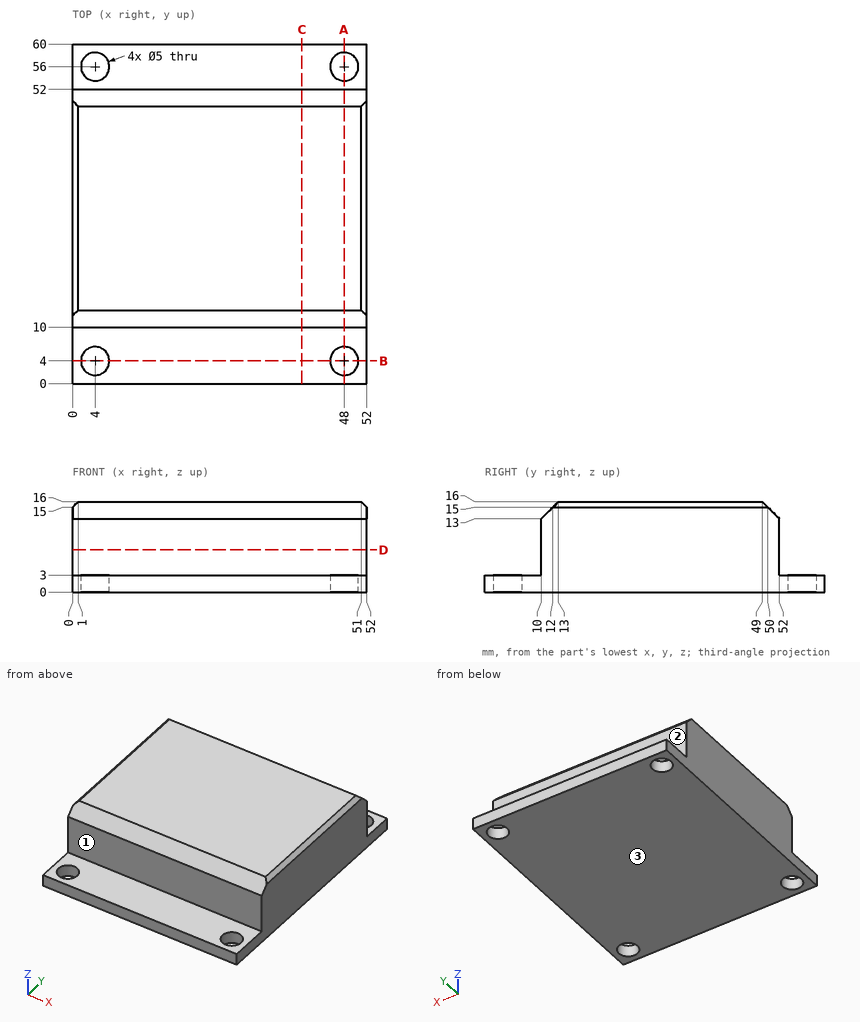
Can you work these out from the drawing? Everything is in mm from the part's minimum corner. A direction names the side the tool comes from. Give positions to 0.01 mm unless a question says otherwise; leave off trailing zeros. Loops run counter-clockwise (first coordinate to the right, second up) from the corner with the lowest first, then second, coordinate; pieces in that order, holes last. Notation, with made-up numbers: M -11.5,46.5 L 24.5,46.5 A26 cw 24.5,62.5 Z; hole C 36,-30 d8. An arc over 180 degrees is marked long. Use CSV: the item, a comma, the result in double quotes. Start each with the question number.
1. On a 3-axis mill with a long thin cutter (end or side, diameter ignored), from which of +Z, -Z, +X, -X, +Y, -Y can I reach the whole of each face in a straight line? I mean the marked faces 1, 2 and 3. Say none if no direction works.
2. Imagine slicing it at D-D, the plane z = 7.5. Write out the boundary of the cut face in (x, y).
3. If I drill on L1, parallel to Y at x = 4, z = 1.75; L2, parallel to Y at x = 27.5, z = 10.75; L3, parallel to Z at x = 46.5, y = 50, over which ranges is the centre line in solid material (lowest first)?
4. Imagine slicing it at C-C, the plane x = 40.5. Write out the boundary of the cut face in (y, z), plus the area to 3 significant figures.
5. Imagine slicing it at A-A, the plane x = 48. Write out the boundary of the cut face in (y, z).
6. Imagine slicing it at B-B, the plane y = 4. Write out the boundary of the cut face in (x, z), plus the area to 3 significant figures.
7. For P1, Ø3, axis at x = 23, y = 3.5, coming from the +Z side; P2, Ø3, axis at x = 36.5, z = 7, coming from the -Y side, each with a flat end and sliding along its axis, tell me the tip position at first contact or that it passes through.
Response values:
1,face 1,"+Z, +X, -X, -Y"
1,face 2,"+Z, +X, -X, +Y"
1,face 3,"-Z, +X, -X, +Y, -Y"
2,outline,"M 0,10 L 52,10 L 52,52 L 0,52 Z"
3,L1,"0 to 1.5, 6.5 to 53.5, 58.5 to 60"
3,L2,"10 to 52"
3,L3,"0 to 15"
4,outline,"M 0,0 L 60,0 L 60,3 L 52,3 L 52,13 L 49,16 L 13,16 L 10,13 L 10,3 L 0,3 Z"
4,area,"717 mm^2"
5,outline,"M 0,0 L 1.5,0 L 1.5,3 L 0,3 Z; M 6.5,0 L 53.5,0 L 53.5,3 L 52,3 L 52,13 L 49,16 L 13,16 L 10,13 L 10,3 L 6.5,3 Z; M 58.5,0 L 60,0 L 60,3 L 58.5,3 Z"
6,outline,"M 0,0 L 1.5,0 L 1.5,3 L 0,3 Z; M 6.5,0 L 45.5,0 L 45.5,3 L 6.5,3 Z; M 50.5,0 L 52,0 L 52,3 L 50.5,3 Z"
6,area,"126 mm^2"
7,P1,"z = 3"
7,P2,"y = 10"
